Study the drawing (mm; zero at the part's minimum x, y, z) and answer. A direction names the side the tool comes from. Give positions to 0.01 mm unless a question says otherwise; leave off trailing zeros. Order: outer loops, then holes, each group sorted by start corner. A loop starts at its lowest first (then second) coordinate and runs counter-clockwise, first axis right, second up.
Item 1: Given pin 1 Ø6.5 at (x, z) = (14, 16) entering from -Y; pin 2 Ø5 at (x, z) = (33, 27) entering from +Y, each flat-ended and moving along its own axis, determine where each tip first touches the part or whether it passes through.
Item 2: A cutting plane is placed at A-A (y = 30). Write down the section's boundary in (x, z), plus the area to 3 significant figures.
Item 3: Find the intervals of material crossed by line 1 along X through (y, z) = (30, 8.25); line 2 along Y through (x, z) = (23, 5.25); line 3 along Y through (x, z) = (23, 12), in increasing order.
Item 4: The mould has two halves that part along Z. Classify the marked faces 1, 2 and 3: +Z half, -Z half, draft (parallel to the pull), parting line (faces both ways), or undercut.
Item 5: Which of the six approach directions +Z, -Z, +X, -X, +Y, -Y give full straight-line access (tool end or side, diameter ignored) to the marked faces 4, 5 and 6?
Item 6: A cutting plane is placed at D-D (y = 37). Write down the section's boundary in (x, z), plus the area to 3 significant figures.
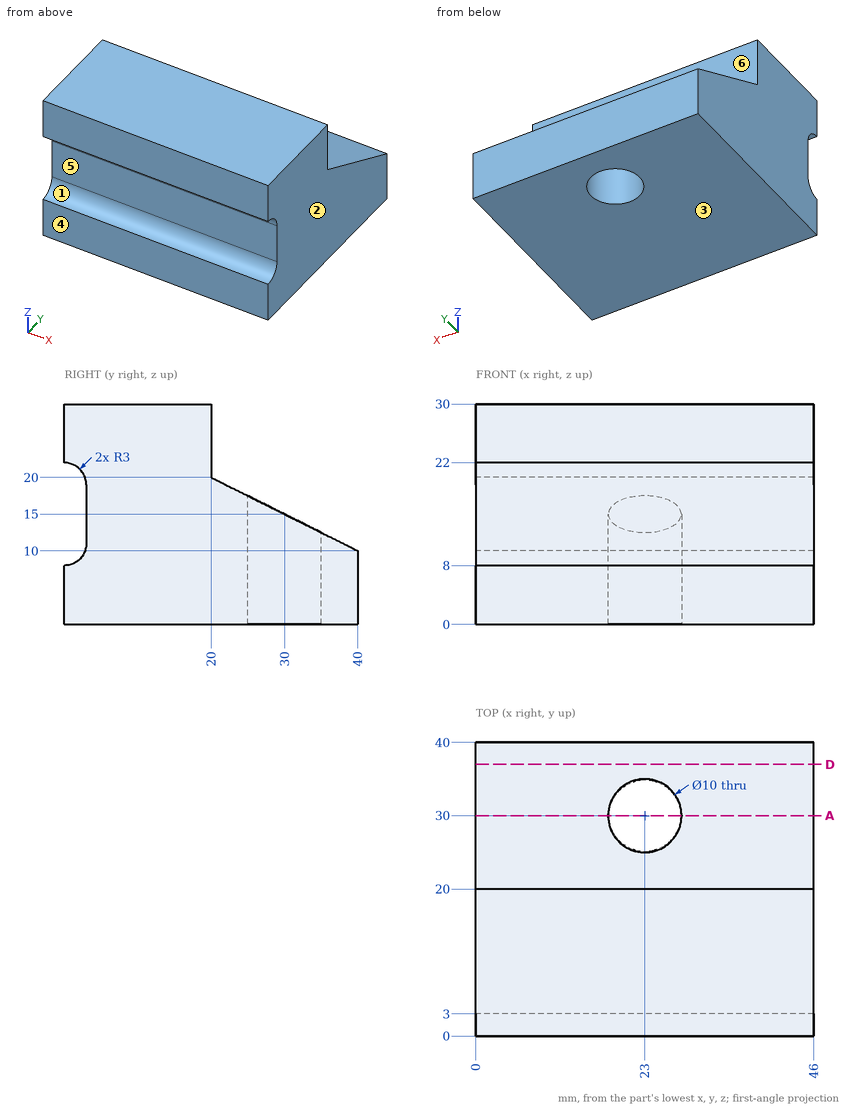
Response values:
1. pin 1: stops at y = 2.99
1. pin 2: stops at y = 20
2. outline: (0, 0) - (18, 0) - (18, 15) - (0, 15) - close; (28, 0) - (46, 0) - (46, 15) - (28, 15) - close
2. area: 540 mm2
3. line 1: x = 0 to 18, 28 to 46
3. line 2: y = 0 to 25, 35 to 40
3. line 3: y = 3 to 25, 35 to 36
4. face 1: undercut
4. face 2: draft
4. face 3: -Z half
5. face 4: +Z, -Z, +X, -X, -Y
5. face 5: +X, -X, -Y
5. face 6: +Z, +X, -X, +Y
6. outline: (0, 0) - (46, 0) - (46, 11.5) - (0, 11.5) - close
6. area: 529 mm2
